```python
from build123d import *

# Parameters (mm, degrees)
SKETCH1_W          = 11.1125
SKETCH1_H          = 3.175
CUT_EXTRUDE2_DEPTH = 2.34696


with BuildPart() as part:
    # Sketch1 → Revolve1 (revolve)
    with BuildSketch(Plane(origin=(0, 0, 0), x_dir=(0, 0, -1), z_dir=(1, 0, 0))):
        with Locations((8.90905, 1.5875)):
            Rectangle(SKETCH1_W, SKETCH1_H)
    revolve(axis=Axis((0, 0, -14.4653), (0, 0, 1)))

    # Sketch7 → Revolve2 (revolve)
    with BuildSketch(Plane(origin=(0, 0, 0), x_dir=(0, 0, -1), z_dir=(1, 0, 0)), mode=Mode.PRIVATE) as revolve2_sk:
        with BuildLine():
            Line((2.84988, 5.5499), (3.3528, 5.5499))
            Line((3.3528, 5.5499), (3.3528, 0))
            Line((3.3528, 0), (0, 0))
            Line((0, 0), (0, 3.175))
            ThreePointArc((0, 3.175), (1.235921075, 4.58927271), (2.84988, 5.5499))
        make_face()
    revolve(revolve2_sk.sketch.rotate(Axis((0, 0, 0), (0, 0, -1)), 180), axis=Axis((0, 0, 0), (0, 0, -1)))

    # Sketch5 → Cut-Extrude2 (cut)
    with BuildSketch(Plane.XY):
        Polygon((1.984375, -1.14567944), (1.984375, 1.14567944), (0, 2.291358881), (-1.984375, 1.14567944), (-1.984375, -1.14567944), (0, -2.291358881), align=None)
    extrude(amount=-CUT_EXTRUDE2_DEPTH, mode=Mode.SUBTRACT)

    # Cut-Extrude3 cone 1 section (through the dimple's axis) → Cut-Extrude3 (revolve, cut)
    with BuildSketch(Plane(origin=(0, 0, 0), x_dir=(0, -1, 0), z_dir=(1, 0, 0))):
        Polygon((0, 0), (2.291358881, 0), (0, 2.291358881), align=None)
    revolve(axis=Axis((0, 0, 0), (0, 0, -1)), mode=Mode.SUBTRACT)


solid = part.part
```
The model under review builds one solid part; all positions refer to its coordinate system, in mm. A direction names the side the tool comes from. Round coordinates to 2 decimals unless told otherwise and drop trailing zeros. Write each loop counter-clockwise with the first axis right and the second up, starting at its lowest first coordinate (ties: lowest second). Pieces come first, ordered by that corner, then holes.
(1) We need section A-A on y = 0. Give the boundary of the cut face in (x, z) (3 decimals).
(2) We need section C-C on z = -11.5. Give the boundary of the cut face in (x, y) (3 decimals).
(3) We need section B-B on z = -1.25. Give the boundary of the cut face in (x, y), and give its area (3 significant figures).
(4) Mouldability with a two-part tool opening along X and no side actions: class faces 1 (the flat face through (-1.984, 0, -1)), 2 (the flat face through (2.4, -2.4, -3.353)), 3 (the cylindrical face through (3.1, -0.69, -8.99)), 4 (the flat face through (1.984, 0, -1)) as +X half, -X half, draft (parallel to the pull), parting line (faces both ways), or undercut.
(5) Insertion check: pin 1 (2 mm diameter, centred on x = 4, y = 2.5, fed in from -Z); pin 2 (1.2 mm diameter, centred on x = -0.5, y = -0.5, fed in from +Z); pin 3 (1 mm diameter, centred on x = 3, y = -2.5, fed in from +Z). Each pin has a flat end and moves straight along its axis. Give the tip position at first contact, or say it passes through.
(6) We need section D-D on x = 4.5. Give the boundary of the cut face in (y, z), and give its area (3 significant figures).
(7) Wall thickness on L1, parallel to X at y = 1.25, z = -2; L2, parallel to X at y = -0.5, z = -3; L3, parallel to Y at x = -3.75, z = -2: over which ranges is each line inside the solid? List them lowest first.
(8) Machinability: for faces 5 (the flat face through (0, 0, -14.465)), 6 (the flat face through (0, 0, -2.347)), which of the approach directions +Z, -Z, +X, -X, +Y, -Y give a long, thin tool a straight path to every point of the face, cutting with its end or side? Answer none if there is none.
Findings below:
1. outline: (-5.55, -3.353) - (-3.175, -3.353) - (-3.175, -14.465) - (3.175, -14.465) - (3.175, -3.353) - (5.55, -3.353) - (5.55, -2.85) arc R5.974 ccw to (3.175, 0) - (2.291, 0) - (1.984, -0.307) - (1.984, -2.347) - (-1.984, -2.347) - (-1.984, -0.307) - (-2.291, 0) - (-3.175, 0) arc R5.974 ccw to (-5.55, -2.85) - close
2. outline: circle Ø6.35 at (0, 0)
3. outline: circle Ø9.2 at (0, 0); hole (-1.98, -1.15) - (0, -2.29) - (1.98, -1.15) - (1.98, 1.15) - (0, 2.29) - (-1.98, 1.15) - close
3. area: 52.9 mm2
4. face 1: undercut
4. face 2: draft
4. face 3: parting line
4. face 4: undercut
5. pin 1: stops at z = -3.35
5. pin 2: stops at z = -2.35
5. pin 3: stops at z = -0.15
6. outline: (-3.25, -3.35) - (3.25, -3.35) - (3.25, -2.85) arc R3.93 ccw to (-3.25, -2.85) - close
6. area: 11.1 mm2
7. L1: x = -4.98 to -1.8, 1.8 to 4.98
7. L2: x = -5.53 to 5.53
7. L3: y = -3.5 to 3.5
8. face 5: -Z, +X, -X, +Y, -Y
8. face 6: +Z
